Source: three-view drawing plus pictorial views. Frame: mm from the lowest corner of the part. A direction names the side the tool comes from. Round coordinates to 2 decimals unless told otherwise and drop trailing zeros. Loops run counter-clockwise (first coordinate to the right, second up) from the corner with the lowest first, then second, coordinate; pieces in that order, holes last. Notation, with made-up numbers: M 29,32.5 L 81,32.5 A21 ccw 81,65.5 Z; hole C 7,33.5 d2. An arc over 180 degrees is marked long. Answer as a JSON object with one key per item and string values.
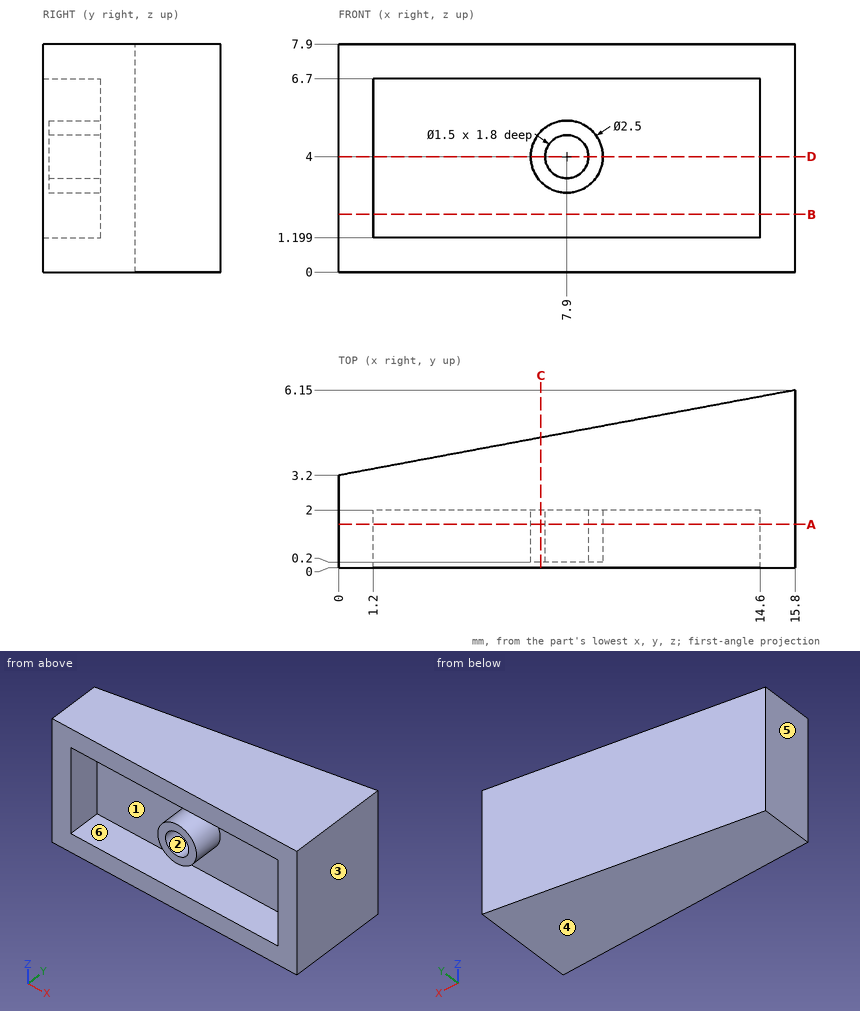
1) Line query: probe 1 along X at (y, z) = (0.9, 4); probe 2 along Z at (x, y) = (7.9, 0.7); probe 3 along Z at (x, y) = (2.25, 0.5). Output: solid intervals per line, ascending.
Geometry results:
{"probe 1": "0 to 1.2, 6.65 to 7.15, 8.65 to 9.15, 14.6 to 15.8", "probe 2": "0 to 1.2, 2.75 to 3.25, 4.75 to 5.25, 6.7 to 7.9", "probe 3": "0 to 1.2, 6.7 to 7.9"}
2) Cut plane A-A on y = 1.5. Return the cut outline in (x, z).
Geometry results:
{"outline": "M 0,0 L 15.8,0 L 15.8,7.9 L 0,7.9 Z; C 7.9,4 d2.5; hole M 1.2,1.2 L 14.6,1.2 L 14.6,6.7 L 1.2,6.7 Z; hole C 7.9,4 d1.5"}
3) First-contact query: pin 1 (3 mm diameter, centred on x = 11.5, z = 3, fed in from -Y); pin 2 (4 mm diameter, centred on x = 3.5, z = 1, fed in from -Y); pin 3 (1.6 mm diameter, centred on x = 8, z = 4, fed in from -Y); pin 4 (1.5 mm diameter, centred on x = 6, z = 4, fed in from +Y). Flat tips, straight axial feed; report the tip coordinate or a pass-through.
Geometry results:
{"pin 1": "y = 2", "pin 2": "y = 0", "pin 3": "y = 0.2", "pin 4": "y = 4.46"}
4) Cut plane B-B on z = 2. Return the cut outline in (x, y), and give its area (3 significant figures).
Geometry results:
{"outline": "M 0,0 L 1.2,0 L 1.2,2 L 14.6,2 L 14.6,0 L 15.8,0 L 15.8,6.15 L 0,3.2 Z", "area": "47.1 mm2"}
5) Pull-direction query (X, two-part tool) for the marked faces 1, 2, 3 and 4; classes: +X half, -X half, draft (parallel to the pull), parting line (faces both ways), or undercut.
Geometry results:
{"face 1": "undercut", "face 2": "undercut", "face 3": "+X half", "face 4": "draft"}
6) Cut plane D-D on z = 4. Return the cut outline in (x, y), and give its area (3 significant figures).
Geometry results:
{"outline": "M 0,0 L 1.2,0 L 1.2,2 L 6.65,2 L 6.65,0.2 L 7.15,0.2 L 7.15,2 L 8.65,2 L 8.65,0.2 L 9.15,0.2 L 9.15,2 L 14.6,2 L 14.6,0 L 15.8,0 L 15.8,6.15 L 0,3.2 Z", "area": "48.9 mm2"}
7) Set-up query: the marked faces 5 and 6. Return all of +Z, -Z, +X, -X, +Y, -Y with unobstructed straight access to the full face (end or side cutting, diameter ignored); none if empty.
Geometry results:
{"face 5": "+Z, -Z, -X, +Y, -Y", "face 6": "-Y"}
8) Cut plane C-C on x = 7. Return the cut outline in (y, z), and give its area (3 significant figures).
Geometry results:
{"outline": "M 0,0 L 4.51,0 L 4.51,7.9 L 0,7.9 L 0,6.7 L 2,6.7 L 2,4.87 L 0.2,4.87 L 0.2,3.13 L 2,3.13 L 2,1.2 L 0,1.2 Z", "area": "27.7 mm2"}
